Could you check a few things on this drawing? It's one solid part, dimensions in mm from its lowest x, y, z. Give positions to 0.01 mm unless a question says otherwise; leave off trailing zeros. Loops run counter-clockwise (first coordinate to the right, second up) from the corner with the lowest first, then second, coordinate; pieces in that order, holes last.
Q1. I need wall thicknesses on probe 1 along Y at (x, z) = (40, 2); probe 2 along Z at (x, y) = (25, 4); probe 3 along Y at (x, z) = (38, 8.5). Which ranges of each line are inside material? Lowest first, please.
Q2. Suppose I cut it at D-D (x = 10). List the corners of the cut face in (y, z) for me.
Q3. Suppose I cut it at B-B (x = 40). List the corners of the cut face in (y, z) for me, and give its area (3 significant figures).
Q4. I'm going to push flat-ended pins straight in: P1, Ø4, axis at y = 3.5, z = 13.5, coming from the -X side; P2, Ø2, axis at y = 3.5, z = 16, coming from the +X side. Where does each tip first touch, or does it pass through?
Q5. Suppose I cut it at A-A (y = 7.5). List the corners of the cut face in (x, z) for me, and give its area (3 significant figures).
Q6. Suppose I cut it at C-C (z = 2.75). List the corners of the cut face in (x, y) for me.
Q7. Thinking about a two-plate mould opening in Y: for the marked faces 1, 2, 3 and 4, which applies, pulls with the +Y half, pulls with the -Y half, needs draft (parallel to the pull), parting line crosses it, or undercut?
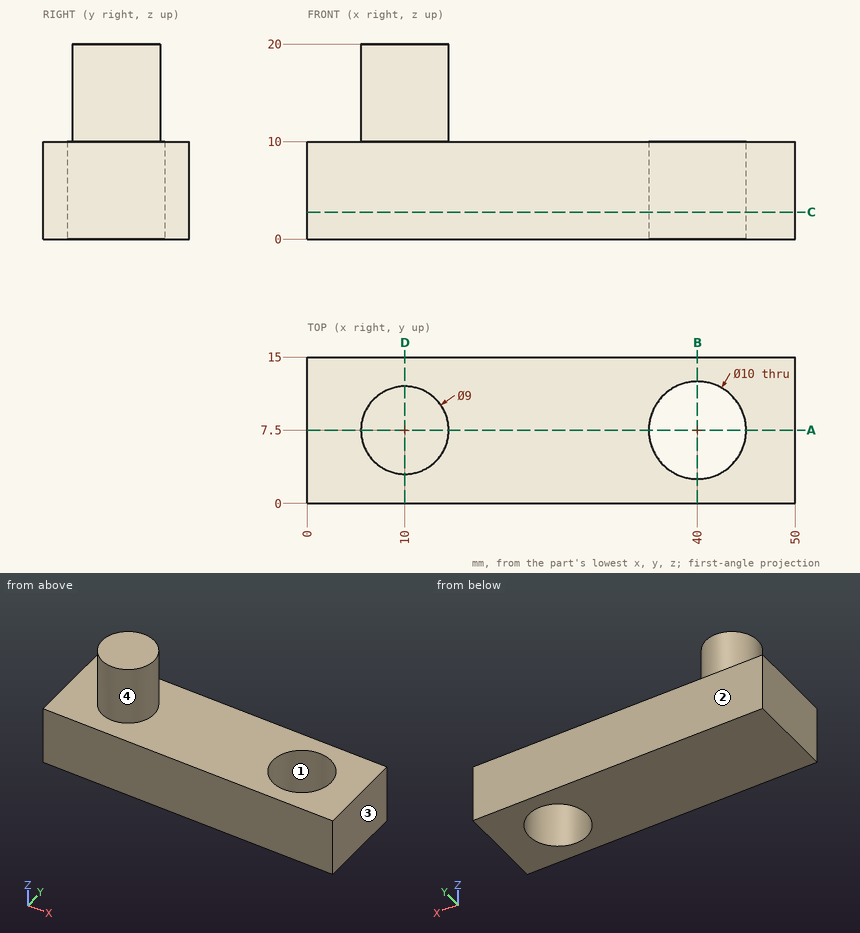
Solutions:
1. probe 1: y = 0 to 2.5, 12.5 to 15
1. probe 2: z = 0 to 10
1. probe 3: y = 0 to 2.92, 12.08 to 15
2. outline: (0, 0) - (15, 0) - (15, 10) - (12, 10) - (12, 20) - (3, 20) - (3, 10) - (0, 10) - close
3. outline: (0, 0) - (2.5, 0) - (2.5, 10) - (0, 10) - close; (12.5, 0) - (15, 0) - (15, 10) - (12.5, 10) - close
3. area: 50.0 mm2
4. P1: stops at x = 5.97
4. P2: stops at x = 13.35
5. outline: (0, 0) - (35, 0) - (35, 10) - (14.5, 10) - (14.5, 20) - (5.5, 20) - (5.5, 10) - (0, 10) - close; (45, 0) - (50, 0) - (50, 10) - (45, 10) - close
5. area: 490 mm2
6. outline: (0, 0) - (50, 0) - (50, 15) - (0, 15) - close; hole circle Ø10 at (40, 7.5)
7. face 1: undercut
7. face 2: pulls with the +Y half
7. face 3: needs draft
7. face 4: parting line crosses it
